Geometry: final body of the model. Coordinates: model frame, mm. Face numbers are marked on the shaded views. Coordinates: 2 decimals unless noted, no trailing zeros. Order: outer loops, then holes, each group sorted by start corner. A loop starts at its lowest first (then second) coordinate and runs counter-clockwise, first axis right, second up. Notation, with made-up numbers: (-15, 34) -> (37, 34) arc R14 cw to (37, 52) -> close; hole circle Ø9 at (-31.5, 38.25). An arc over 180 degrees is marked (long way). Use CSV: the item, a comma, the result in double quotes. Start each with the question number.
from build123d import *

# Parameters (mm, degrees)
SCHIZZO1_R                                    = 14
SCHIZZO1_R_2                                  = 8
ESTRUSIONE_ESTRUSIONE1_DEPTH                  = 20
ESTRUSIONE_ESTRUSIONE2_REACH                  = 30.142
ESTRUSIONE_ESTRUSIONE2_END_RADIUS             = 14
SCHIZZO2_W                                    = 45
SCHIZZO2_H                                    = 28
ESTRUSIONE_ESTRUSIONE2_DIRECTION_2_REACH      = 30.142
ESTRUSIONE_ESTRUSIONE2_DIRECTION_2_END_RADIUS = 14


with BuildPart() as part:
    # Schizzo1 → Estrusione-Estrusione1 (new body)
    with BuildSketch(Plane.XY):
        Circle(SCHIZZO1_R)
        Circle(SCHIZZO1_R_2, mode=Mode.SUBTRACT)
    extrude(amount=ESTRUSIONE_ESTRUSIONE1_DEPTH)

    # Estrusione-Estrusione2: up to this cylinder (the profile starts inside it)
    estrusione_estrusione2_end = Plane(origin=(0, 0, -22.5), z_dir=(0, 0, -1)) * Cylinder(ESTRUSIONE_ESTRUSIONE2_END_RADIUS, 89.284, mode=Mode.PRIVATE)
    # Schizzo2 → Estrusione-Estrusione2 (add, up to the surface)
    with BuildSketch(Plane(origin=(0, 0, 0), x_dir=(0, 0, -1), z_dir=(1, 0, 0)), mode=Mode.PRIVATE) as estrusione_estrusione2_sk1:
        with Locations((22.5, 0)):
            Rectangle(SCHIZZO2_W, SCHIZZO2_H)
        with BuildLine():
            Line((35, -2.5), (10, -2.5))
            ThreePointArc((10, -2.5), (7.5, 0), (10, 2.5))
            Line((10, 2.5), (35, 2.5))
            ThreePointArc((35, 2.5), (37.5, 0), (35, -2.5))
        make_face(mode=Mode.SUBTRACT)
    estrusione_estrusione2_tool1 = extrude(estrusione_estrusione2_sk1.sketch, amount=ESTRUSIONE_ESTRUSIONE2_REACH, mode=Mode.PRIVATE) & estrusione_estrusione2_end
    add(estrusione_estrusione2_tool1.solids().sort_by_distance((0, -13.47, -22.5))[0])

    # Estrusione-Estrusione2 direction 2: up to this cylinder (the profile starts inside it)
    estrusione_estrusione2_direction_2_end = Plane(origin=(0, 0, -22.5), z_dir=(0, 0, -1)) * Cylinder(ESTRUSIONE_ESTRUSIONE2_DIRECTION_2_END_RADIUS, 89.284, mode=Mode.PRIVATE)
    # Schizzo2 → Estrusione-Estrusione2 direction 2 (add, up to the surface)
    with BuildSketch(Plane(origin=(0, 0, 0), x_dir=(0, 0, -1), z_dir=(1, 0, 0)), mode=Mode.PRIVATE) as estrusione_estrusione2_direction_2_sk1:
        with Locations((22.5, 0)):
            Rectangle(SCHIZZO2_W, SCHIZZO2_H)
        with BuildLine():
            Line((35, -2.5), (10, -2.5))
            ThreePointArc((10, -2.5), (7.5, 0), (10, 2.5))
            Line((10, 2.5), (35, 2.5))
            ThreePointArc((35, 2.5), (37.5, 0), (35, -2.5))
        make_face(mode=Mode.SUBTRACT)
    estrusione_estrusione2_direction_2_tool1 = extrude(estrusione_estrusione2_direction_2_sk1.sketch, amount=-ESTRUSIONE_ESTRUSIONE2_DIRECTION_2_REACH, mode=Mode.PRIVATE) & estrusione_estrusione2_direction_2_end
    add(estrusione_estrusione2_direction_2_tool1.solids().sort_by_distance((0, -13.47, -22.5))[0])


solid = part.part
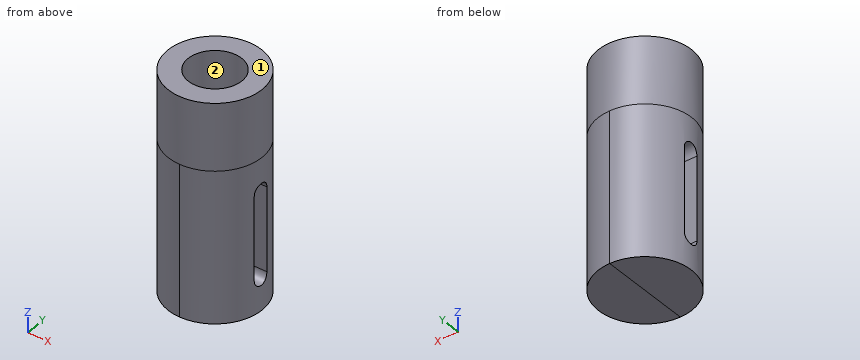
(1) Mould query, pull axis X, two halves, no side actions, for the marked faces 1 and 2. Classes: pulls with the +X half, pulls with the -X half, needs draft (parallel to the pull), parting line crosses it, or undercut.
(2) First-contact query: pin 1 (4 mm diameter, centred on y = 11, z = -6, fed in from +X); pin 2 (1.5 mm diameter, centred on x = -7, z = -19.5, fed in from +Y); pin 3 (8 mm diameter, centred on x = -8, z = -33.5, fed in from +Y). Flat tips, straight axial feed; report the tip coordinate or a pass-through.
(3) Section A-A (y = 1.75). Return loops of the section in (x, z).
(4) Section D-D (z = 1). Return loops of the section in (x, y).
(5) Section C-C (x = -11). Return loops of the section in (y, z).
(6) Section B-B (z = -27). Return loops of the section in (x, y), then the cut area to 4 significant figures.
(7) Line query: line 1 (Y direction, x = 0, z = 7.25); line 2 (X direction, y = -0.5, z = 2); line 3 (Z direction, x = -9.25, y = -0.25). Output: solid intervals per line, ascending. Write a range as from..to.
Check sheet entries:
1,face 1,"needs draft"
1,face 2,"undercut"
2,pin 1,"stops at x = 10.72"
2,pin 2,"stops at y = 12.53"
2,pin 3,"stops at y = 13.42"
3,outline,"(-13.89, -45) -> (13.89, -45) -> (13.89, -36.79) -> (-13.89, -36.79) -> close; (-13.89, -8.21) -> (13.89, -8.21) -> (13.89, 20) -> (7.81, 20) -> (7.81, 0) -> (-7.81, 0) -> (-7.81, 20) -> (-13.89, 20) -> close"
4,outline,"circle Ø28 at (0, 0); hole circle Ø16 at (0, 0)"
5,outline,"(-8.66, -45) -> (8.66, -45) -> (8.66, 20) -> (-8.66, 20) -> close; hole (-2.5, -35) arc R2.5 ccw to (2.5, -35) -> (2.5, -10) arc R2.5 ccw to (-2.5, -10) -> close"
6,outline,"(-13.77, -2.5) arc R14 ccw to (13.77, -2.5) -> close; (-13.77, 2.5) -> (13.77, 2.5) arc R14 ccw to start"
6,area,"476.5 mm^2"
7,line 1,"y = -14..-8, 8..14"
7,line 2,"x = -13.99..-7.98, 7.98..13.99"
7,line 3,"z = -45..-37.49, -7.51..20"
